```python
from build123d import *

# Parameters (mm, degrees)
SKETCH1_R           = 64
SKETCH1_R_2         = 5
BOSS_EXTRUDE1_DEPTH = 10
SKETCH2_R           = 15
BOSS_EXTRUDE2_DEPTH = 7
SKETCH3_R           = 10
CUT_EXTRUDE1_DEPTH  = 10
FILLET1_R           = 10
CHAMFER1_SIZE       = 7


with BuildPart() as part:
    # Sketch1 → Boss-Extrude1 (new body)
    with BuildSketch(Plane.XY):
        Circle(SKETCH1_R)
        Circle(SKETCH1_R_2, mode=Mode.SUBTRACT)
    extrude(amount=BOSS_EXTRUDE1_DEPTH)

    # Sketch2 → Boss-Extrude2 (add)
    with BuildSketch(Plane.XY.offset(10)):
        Circle(SKETCH2_R)
        Polygon((7.505553499, 0), (3.75277675, 6.5), (-3.75277675, 6.5), (-7.505553499, 0), (-3.75277675, -6.5), (3.75277675, -6.5), align=None, mode=Mode.SUBTRACT)
    extrude(amount=BOSS_EXTRUDE2_DEPTH)

    # Sketch3 → Cut-Extrude1 (cut)
    with BuildSketch(Plane(origin=(0, 0, 0), x_dir=(-1, 0, 0), z_dir=(0, 0, -1))):
        with Locations((56.533626817, 32.077235525)):
            Circle(SKETCH3_R)
        with Locations((32.077235525, -56.533626817)):
            Circle(SKETCH3_R)
        with Locations((-56.533626817, -32.077235525)):
            Circle(SKETCH3_R)
        with Locations((-32.077235525, 56.533626817)):
            Circle(SKETCH3_R)
    extrude(amount=-CUT_EXTRUDE1_DEPTH, mode=Mode.SUBTRACT)

    # Fillet1
    fillet1_edges = [part.edges().sort_by_distance(p)[0] for p in [
        (22.646447987, 59.859321693, 5),
        (39.769398937, 50.143742463, 5),
        (59.859321693, -22.646447987, 5),
        (50.143742463, -39.769398937, 5),
        (-22.646447987, -59.859321693, 5),
        (-39.769398937, -50.143742463, 5),
        (-59.859321693, 22.646447987, 5),
        (-50.143742463, 39.769398937, 5),
    ]]
    fillet(fillet1_edges, radius=FILLET1_R)

    # Chamfer1
    chamfer1_edges = [part.edges().sort_by_distance(p)[0] for p in [
        (-15, 0, 10),
    ]]
    chamfer(chamfer1_edges, length=CHAMFER1_SIZE - 0.0001)  # a hair under: the kernel refuses the full size

    # Fillet2: read off the stored shape, not the designer's step
    # Fillet2 outline → Fillet2 (revolve, cut)
    with BuildSketch(Plane.XZ):
        with BuildLine():
            ThreePointArc((12.928932188, 17), (14.84234935, 16.619397663), (16.464466094, 15.535533906))
            Line((16.464466094, 15.535533906), (16.464466094, 17))
            Line((16.464466094, 17), (12.928932188, 17))
        make_face()
    revolve(axis=Axis((0, 0, 0), (0, 0, 1)), mode=Mode.SUBTRACT)

    # Fillet2 2 outline → Fillet2 2 (revolve)
    with BuildSketch(Plane.XZ):
        with BuildLine():
            ThreePointArc((24.071067812, 10), (22.15765065, 10.380602337), (20.535533906, 11.464466094))
            Line((20.535533906, 11.464466094), (20.535533906, 10))
            Line((20.535533906, 10), (24.071067812, 10))
        make_face()
    revolve(axis=Axis((0, 0, 0), (0, 0, 1)))


solid = part.part
```
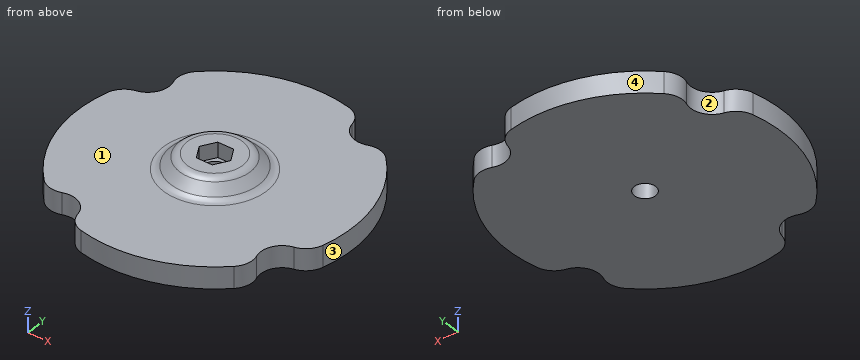
Geometry check sheet. Reference: the model listing, model coordinates, mm. Face numbers are marked on the shaded views. Coordinates: 2 decimals unless noted, no trailing zeros. Loops run counter-clockwise (first coordinate to the right, second up) from the corner with the lowest first, then second, coordinate; pieces in that order, holes last. Notation, with made-up numbers: (-7.5, 17.25) - (29.5, 17.25) arc R14 ccw to (29.5, 26.25) - close; hole circle Ø5 at (36.25, -9). An arc over 180 degrees is marked (long way). One line per item, written item: value. Start each with the question number.
(1) Cross-section at C-C on x = -53. Enter the section's corners in (y, z).
(2) Mould release check, pull along Y, two halves, no side actions. Record for the marked faces 1, 2, 3 and 4: released by +Y, released by -Y, zero draft, split by the parting line, or undercut.
(3) Depth check by flat-ended pin: P1, Ø6, axis at x = -21.5, z = 3, coming from the +Y side; P2, Ø6.5, axis at x = -3, y = -0.5, coming from the +Z side; P3, Ø8, axis at x = -8.5, z = 6, coming from the -Y side; P4, Ø3, axis at x = -47.5, z = 13, coming from the -Y side. Enter the tip coordinate at first touch or a pass-through.
(4) Material ranges on line 1 (X direction, y = 0, z = 11.5); line 2 (Z direction, x = -31.5, y = 4.5); line 3 (Y direction, x = 0, z = 4), recorded low to high. Write a range as [from, to].
(5) Cross-section at B-B on x = -26. Enter the section's corners in (y, z).
Results below:
1. outline: (-35.87, 0) - (22.72, 0) - (22.72, 10) - (-35.87, 10) - close
2. face 1: zero draft
2. face 2: undercut
2. face 3: split by the parting line
2. face 4: released by +Y
3. P1: stops at y = 61.27
3. P2: stops at z = 10
3. P3: stops at y = -63.84
3. P4: passes through
4. line 1: x = [-20.5, -7.51], [7.51, 20.5]
4. line 2: z = [0, 10]
4. line 3: y = [-64, -5], [5, 64]
5. outline: (-48.59, 0) - (58.48, 0) - (58.48, 10) - (-48.59, 10) - close
